Print and shaded views of the part. All mm, measured from the part's lowest x, y and z. A direction names the side the tool comes from. Give positions to 0.01 mm unless a question says otherwise; leave off trailing zeros. Loops run counter-clockwise (first coordinate to the right, second up) from the corner with the lowest first, then second, coordinate; pieces in that order, holes last.
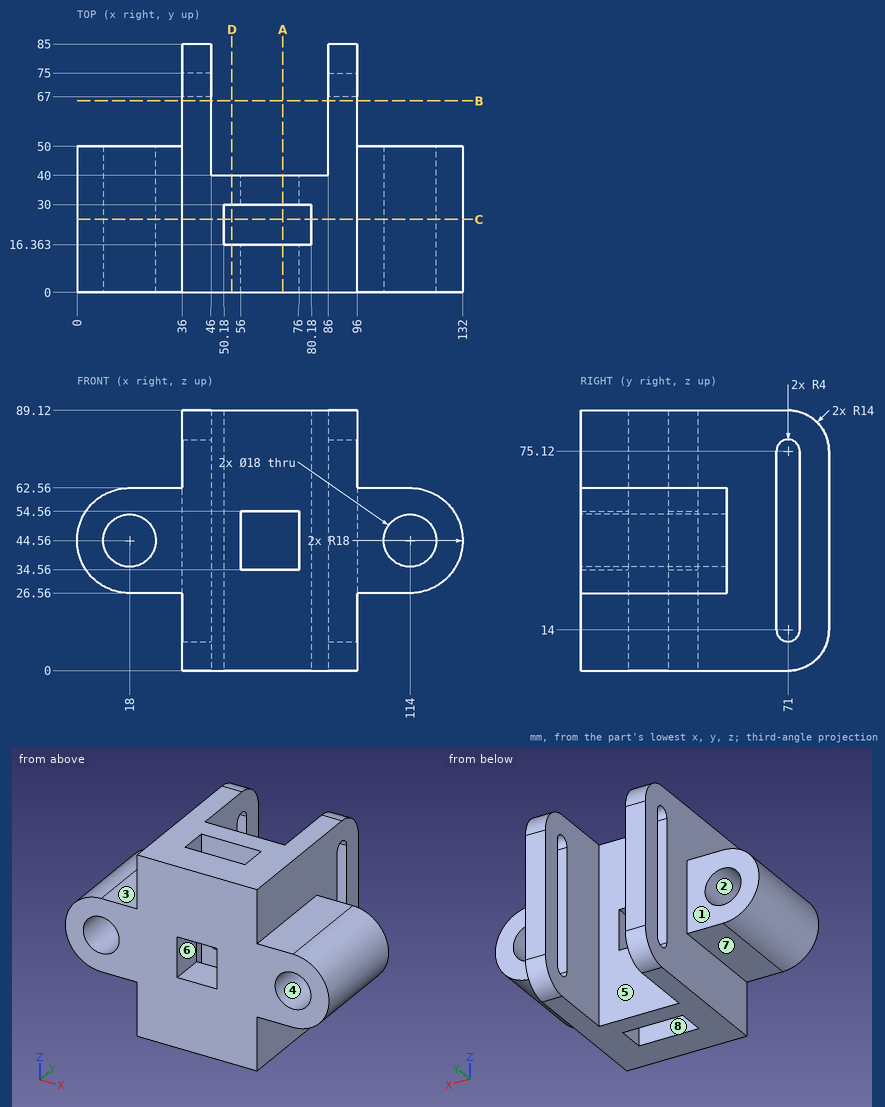
1. Probe line 1 along X through (y, z) = (13, 44); line 2 along X through (y, z) = (63, 80.5); line 3 along X through (y, z) = (29, 44). List the from-to ranges inside material, lowest first.
Responses:
line 1: x = 0.01 to 9.02, 26.98 to 56, 76 to 105.02, 122.98 to 131.99
line 2: x = 36 to 46, 86 to 96
line 3: x = 0.01 to 9.02, 26.98 to 50.18, 80.18 to 105.02, 122.98 to 131.99
2. Drop flat-ended pins along their axis: pin 1 (22.5 mm diameter, centred on y = 61.5, z = 47, fed in from +X); pin 2 (12 mm diameter, centred on x = 112.5, z = 45.5, fed in from -Y); pin 3 (3 mm diameter, centred on y = 35, z = 40, fed in from +X); pin 4 (9 mm diameter, centred on x = 107, y = 20.5, fed in from -Z). Give the stop position or say it passes through.
Responses:
pin 1: stops at x = 96
pin 2: passes through
pin 3: stops at x = 131.74
pin 4: stops at z = 26.56
3. Tool access for the marked faces 5, 6, 7 and 8: list every direction of +Z, -Z, +X, -X, +Y, -Y with a clear straight run to the whole face (end or side of a thin tool).
Responses:
face 5: +Z, -Z, +Y
face 6: +Y, -Y
face 7: -Z, -X, +Y, -Y
face 8: +Z, -Z
4. Saw through at B-B, the plane y = 65.5. List the corners of the cut face in (x, z), and give its area (3 significant figures).
Responses:
outline: (36, 0) - (46, 0) - (46, 89.12) - (36, 89.12) - close; (86, 0) - (96, 0) - (96, 89.12) - (86, 89.12) - close
area: 1,780 mm2
5. Saw through at D-D, the plane x = 53. List the corners of the cut face in (y, z), and give its area (3 significant figures).
Responses:
outline: (0, 0) - (16.36, 0) - (16.36, 89.12) - (0, 89.12) - close; (30, 0) - (40, 0) - (40, 89.12) - (30, 89.12) - close
area: 2,350 mm2
6. Saw through at C-C, the plane y = 25. List the corners of the cut face in (x, z), and give its area (3 significant figures).
Responses:
outline: (18, 26.56) - (36, 26.56) - (36, 0) - (50.18, 0) - (50.18, 89.12) - (36, 89.12) - (36, 62.56) - (18, 62.56) arc R18 ccw to start; (80.18, 0) - (96, 0) - (96, 26.56) - (114, 26.56) arc R18 ccw to (114, 62.56) - (96, 62.56) - (96, 89.12) - (80.18, 89.12) - close; hole circle Ø18 at (18, 44.56); hole circle Ø18 at (114, 44.56)
area: 4,480 mm2
7. Saw through at A-A, the plane x = 70.5. List the corners of the cut face in (y, z).
Responses:
outline: (0, 0) - (16.36, 0) - (16.36, 34.56) - (0, 34.56) - close; (0, 54.56) - (16.36, 54.56) - (16.36, 89.12) - (0, 89.12) - close; (30, 0) - (40, 0) - (40, 34.56) - (30, 34.56) - close; (30, 54.56) - (40, 54.56) - (40, 89.12) - (30, 89.12) - close
8. Pull direction Z, two halves, no side cores. Call the marked faces 1, 2, 3 and 4: released by +Z, released by -Z, zero draft, split by the parting line, or undercut.
Responses:
face 1: zero draft
face 2: undercut
face 3: released by +Z
face 4: undercut
